Autodesk Inventor part; units mm, degrees
ref_plane "YZ Plane" through (0, 0, 0) normal (1, 0, 0) x (0, 1, 0)
ref_plane "XZ Plane" through (0, 0, 0) normal (0, 1, 0) x (-1, 0, 0)
ref_plane "XY Plane" through (0, 0, 0) normal (0, 0, 1) x (1, 0, 0)
sketch "Sketch1" plane through (0, 0, 0) normal (0, 0, 1) x (1, 0, 0)
  line L0 (0, 0) -> (71, 0)
  line L1 (71, 0) -> (71, -150)
  line L2 (71, -150) -> (0, -150)
  line L3 (0, -150) -> (0, 0)
  line L4 (7.6868, 0) -> (92.3291, 0)
  line L5 (9.7325, -150) -> (92.3291, -150)
  line L6 (9.7325, -150) -> (11.7224, -150)
  line L7 (0, 0) -> (5, -5)
  line L8 (0, 0) -> (7.0711, 0) construction
  line L9 (5, -5) -> (0, -10)
  line L10 (0, -10) -> (5, -15)
  line L11 (5, -15) -> (0, -20)
  line L12 (0, -20) -> (5, -25)
  line L13 (5, -25) -> (0, -30)
  line L14 (0, -30) -> (5, -35)
  line L15 (5, -35) -> (0, -40)
  line L16 (0, -40) -> (5, -45)
  line L17 (5, -45) -> (0, -50)
  line L18 (0, -50) -> (5, -55)
  line L19 (5, -55) -> (0, -60)
  line L20 (0, -60) -> (5, -65)
  line L21 (5, -65) -> (0, -70)
  line L22 (0, -70) -> (5, -75)
  line L23 (5, -75) -> (0, -80)
  line L24 (0, -80) -> (5, -85)
  line L25 (5, -85) -> (0, -90)
  line L26 (0, -90) -> (5, -95)
  line L27 (5, -95) -> (0, -100)
  line L28 (0, -100) -> (5, -105)
  line L29 (5, -105) -> (0, -110)
  line L30 (0, -110) -> (5, -115)
  line L31 (5, -115) -> (0, -120)
  line L32 (0, -120) -> (5, -125)
  line L33 (5, -125) -> (0, -130)
  line L34 (0, -130) -> (5, -135)
  line L35 (5, -135) -> (0, -140)
  line L36 (35.5, 0) -> (35.5, -140) construction
  line L37 (71, 0) -> (66, -5)
  line L38 (66, -5) -> (71, -10)
  line L39 (71, -10) -> (66, -15)
  line L40 (66, -15) -> (71, -20)
  line L41 (71, -20) -> (66, -25)
  line L42 (66, -25) -> (71, -30)
  line L43 (71, -30) -> (66, -35)
  line L44 (66, -35) -> (71, -40)
  line L45 (71, -40) -> (66, -45)
  line L46 (66, -45) -> (71, -50)
  line L47 (71, -50) -> (66, -55)
  line L48 (66, -55) -> (71, -60)
  line L49 (71, -60) -> (66, -65)
  line L50 (66, -65) -> (71, -70)
  line L51 (71, -70) -> (66, -75)
  line L52 (66, -75) -> (71, -80)
  line L53 (71, -80) -> (66, -85)
  line L54 (66, -85) -> (71, -90)
  line L55 (71, -90) -> (66, -95)
  line L56 (66, -95) -> (71, -100)
  line L57 (71, -100) -> (66, -105)
  line L58 (66, -105) -> (71, -110)
  line L59 (71, -110) -> (66, -115)
  line L60 (66, -115) -> (71, -120)
  line L61 (71, -120) -> (66, -125)
  line L62 (66, -125) -> (71, -130)
  line L63 (71, -130) -> (66, -135)
  line L64 (66, -135) -> (71, -140)
  line L65 (10, -3) -> (61, -3)
  line L66 (61, -3) -> (61, -6)
  line L67 (61, -6) -> (10, -6)
  line L68 (10, -6) -> (10, -3)
  line L69 (10, -144) -> (61, -144)
  line L70 (61, -144) -> (61, -147)
  line L71 (61, -147) -> (10, -147)
  line L72 (10, -147) -> (10, -144)
  line L73 (0, -140) -> (5, -145)
  line L74 (5, -145) -> (0, -150)
  line L75 (66, -5) -> (71, -10)
  line L76 (71, -140) -> (66, -145)
  line L77 (66, -145) -> (71, -150)
  line L78 (11, -80) -> (11, -140) construction
  line L79 (9.4, -80) -> (9.4, -140)
  line L80 (12.6, -140) -> (12.6, -80)
  arc A0 (12.6, -80) -> (9.4, -80) centre (11, -80) ccw
  arc A1 (9.4, -140) -> (12.6, -140) centre (11, -140) ccw
  line L81 (16.5, -40) -> (16.5, -60) construction
  line L82 (15, -40) -> (15, -60)
  line L83 (18, -60) -> (18, -40)
  arc A2 (18, -40) -> (15, -40) centre (16.5, -40) ccw
  arc A3 (15, -60) -> (18, -60) centre (16.5, -60) ccw
  line L84 (54.5, -40) -> (54.5, -60) construction
  line L85 (56, -40) -> (56, -60)
  line L86 (53, -60) -> (53, -40)
  arc A4 (56, -40) -> (53, -40) centre (54.5, -40) ccw
  arc A5 (53, -60) -> (56, -60) centre (54.5, -60) ccw
  line L87 (60, -80) -> (60, -140) construction
  line L88 (61.6, -80) -> (61.6, -140)
  line L89 (58.4, -140) -> (58.4, -80)
  arc A6 (61.6, -80) -> (58.4, -80) centre (60, -80) ccw
  arc A7 (58.4, -140) -> (61.6, -140) centre (60, -140) ccw
  line L90 (35.5, -129) -> (35.5, -94) construction
  line L91 (43, -129) -> (43, -94)
  line L92 (28, -94) -> (28, -129)
  arc A8 (28, -129) -> (43, -129) centre (35.5, -129) ccw
  arc A9 (43, -94) -> (28, -94) centre (35.5, -94) ccw
  line L93 (35.5, -56) -> (35.5, -21) construction
  line L94 (43, -56) -> (43, -21)
  line L95 (28, -21) -> (28, -56)
  arc A10 (28, -56) -> (43, -56) centre (35.5, -56) ccw
  arc A11 (43, -21) -> (28, -21) centre (35.5, -21) ccw
  line L96 (71, -75) -> (0, -75) construction
  line L97 (11, -70) -> (11, -10) construction
  line L98 (9.4, -70) -> (9.4, -10)
  line L99 (12.6, -10) -> (12.6, -70)
  arc A12 (9.4, -70) -> (12.6, -70) centre (11, -70) ccw
  arc A13 (12.6, -10) -> (9.4, -10) centre (11, -10) ccw
  line L100 (61.6, -70) -> (61.6, -10)
  line L101 (58.4, -10) -> (58.4, -70)
  line L102 (60, -70) -> (60, -10) construction
  arc A14 (61.6, -10) -> (58.4, -10) centre (60, -10) ccw
  arc A15 (58.4, -70) -> (61.6, -70) centre (60, -70) ccw
  point P0 (11, -110)
  point P1 (16.5, -50)
  point P2 (54.5, -50)
  point P3 (60, -110)
  point P4 (35.5, -111.5)
  point P5 (35.5, -38.5)
  point P6 (11, -40)
  point P7 (60, -40)
  dimension "d0" = 71
  dimension "d1" = 150
  dimension "d2" = 45
  dimension "d3" = 5
  dimension "d6" = 10
  dimension "d11" = 35.5
  dimension "d12" = 10
  dimension "d13" = 10
  dimension "d14" = 3
  dimension "d15" = 10
  dimension "d16" = 3
  dimension "d17" = 138
  dimension "d19" = 6
  dimension "d20" = 3.2
  dimension "d21" = 11
  dimension "d22" = 10
  dimension "d24" = 51
  dimension "d25" = 3
  dimension "d26" = 4
  dimension "d27" = 40
  dimension "d28" = 20
  dimension "d29" = 35
  dimension "d30" = 41
  dimension "d36" = 35
  dimension "d37" = 15
  dimension "d38" = 15
  dimension "d39" = 35
  dimension "d40" = 15
  dimension "d41" = 15
  dimension "d44" = 60
  dimension "d45" = 75
extrude "Extrusion1" add sketch "Sketch1" along normal blind 2.5 contours L0 L37 L38 L39 L40 L41 L42 L43 L44 L45 L46 L47 L48 L49 L50 L51 L52 L53 L54 L55 L56 L57 L58 L59 L60 L61 L62 L63 L64 L76 L77 L2 L74 L73 L35 L34 L33 L32 L31 L30 L29 L28 L27 L26 L25 L24 L23 L22 L21 L20 L19 L18 L17 L16 L15 L14 L13 L12 L11 L10 L9 L7 | L65 L66 L67 L68 | L69 L70 L71 L72 | A8 L92 A9 L91 | A10 L95 A11 L94 | L98 A13 L99 A12 | A15 L101 A14 L100
extrude "Extrusion2" add sketch "Sketch1" along normal blind 8 contours L65 L66 L67 L68 | L69 L70 L71 L72
fillet "Fillet1" radius 3 2 edges at (35.5, -147, 2.5) (35.5, -3, 2.5)
extrude "Extrusion3" cut sketch "Sketch1" along normal through all contours A8 L92 A9 L91 | A10 L95 A11 L94
extrude "Extrusion4" cut sketch "Sketch1" along normal through all contours L98 A13 L99 A12 | A15 L101 A14 L100
equation "\"d11\" = 0.5 * d0"
equation "\"d13\" = d12"
equation "\"d15\" = d12"
equation "\"d16\" = d14"
equation "\"d19\" = -0.5 * d17 + 0.5 * d1"
equation "\"d45\" = 0.5 * d1"
properties part number "tray"
Build history of the part. All positions in model axes, mm. A direction names the side the tool comes from. Round coordinates to 2 decimals unless told otherwise and drop trailing zeros. Order: outer loops, then holes, each group sorted by start corner. A loop starts at its lowest first (then second) coordinate and runs counter-clockwise, first axis right, second up. Notation, with made-up numbers: (3.5, 9.25) -> (40.5, 9.25) arc R31 ccw to (40.5, 47.25) -> close; hole circle Ø10 at (-11, -3). An arc over 180 degrees is marked (long way). Answer in a Markdown table with one row per item.
1) Band-saw the part on C-C on y = -132. Give the cut face in (x, z), and give its area (3 significant figures).
Values:
| item | result |
|---|---|
| outline | (2, 0) -> (9.4, 0) -> (9.4, 2.5) -> (2, 2.5) -> close; (12.6, 0) -> (28.63, 0) -> (28.63, 2.5) -> (12.6, 2.5) -> close; (42.37, 0) -> (58.4, 0) -> (58.4, 2.5) -> (42.37, 2.5) -> close; (61.6, 0) -> (69, 0) -> (69, 2.5) -> (61.6, 2.5) -> close |
| area | 117 mm2 |
2) Which spindle directions (+Z, -Z, +X, -X, +Y, -Y) get a long thin tool onto all of the face, cutting with end or side? Do faces 5 (the cylindrical face through (35.86, -147.9, 3.36)), 6 (the flat face through (69, -122, 1)), 7 (the flat face through (35, -3, 7)), 8 (the flat face through (9.4, -110, 1)), 9 (the flat face through (2, -12, 1)). Say none if no direction does.
Values:
| item | result |
|---|---|
| face 5 | +Z, +X, -X, -Y |
| face 6 | +Z, -Z, +X |
| face 7 | +Z, +X, -X, +Y |
| face 8 | +Z, -Z |
| face 9 | +Z, -Z, -X |
3) Mould opens along X. For faces 1 (the flat face through (3, -147, 1)), 2 (the flat face through (68, -27, 1)), 3 (the cylindrical face through (35.34, -13.5, 1.23)), 4 (the flat face through (61.6, -110, 1)) say: released by +X, released by -X, zero draft, split by the parting line, or undercut.
Values:
| item | result |
|---|---|
| face 1 | released by -X |
| face 2 | released by +X |
| face 3 | undercut |
| face 4 | undercut |
4) Wall check: L1, parallel to Y at x = 60, z = 1; L2, parallel to Y at x = 38, z = 5.5; L3, parallel to X at y = -60.5, z = 1.25. Give the ranges that are in metal, low to high.
Values:
| item | result |
|---|---|
| L1 | -150 to -141.6, -78.4 to -71.6, -8.4 to 0 |
| L2 | -147 to -144, -6 to -3 |
| L3 | 0.5 to 9.4, 12.6 to 15.09, 17.91 to 29.5, 41.5 to 53.09, 55.91 to 58.4, 61.6 to 70.5 |
5) Pin check, flat tips, straight feed: P1, Ø2, axis at x = 24, y = -86, coming from the +Z side; P2, Ø2, axis at y = -32, z = 2.5, coming from the +X side; P3, Ø3, axis at y = -40.5, z = 1.5, coming from the -X side; P4, Ø4.5, axis at x = 46.5, z = 6, coming from the -Y side. Stop position of each tip, or through.
Values:
| item | result |
|---|---|
| P1 | z = 2.5 |
| P2 | x = 70 |
| P3 | x = 0 |
| P4 | y = -147.56 |
6) Band-saw the part on B-B on x = 35.5. Give the number of separate pieces and of enclosed holes in the cut face, and give its area (3 significant figures).
Values:
| item | result |
|---|---|
| separate pieces | 3 |
| enclosed holes | 0 |
| area | 162 mm2 |
